Check sheet for the modelled part. Datum: model origin and axes. Units: mm. Face numbers are marked on the shaded views. A direction names the side the tool comes from. Give positions to 0.01 mm unless a question says otherwise; leave off trailing zeros. Write each loop counter-clockwise with the first axis right and the second up, starting at its lowest first coordinate (ties: lowest second). Pieces come first, ordered by that corner, then holes. Notation, with made-up numbers: (49.5, -1) - (59.5, -1) arc R15 cw to (59.5, 27) - close; hole circle Ø1 at (-23, 80). An arc over 180 degrees is marked (long way). Return JSON: item names as keys, results as strings. Group by question number.
```python
from build123d import *

# Parameters (mm, degrees)
SKETCH1_W           = 82.55
SKETCH1_H           = 22.225
BOSS_EXTRUDE1_DEPTH = 6.35
SKETCH3_W           = 3.175
SKETCH3_H           = 25.4
BOSS_EXTRUDE2_DEPTH = 22.225
CUT_EXTRUDE3_START  = 3.175
SKETCH2_W           = 38.1
SKETCH2_H           = 3.175
CUT_EXTRUDE3_DEPTH  = 50.972604439


with BuildPart() as part:
    # Sketch1 → Boss-Extrude1 (new body)
    with BuildSketch(Plane.XY):
        Rectangle(SKETCH1_W, SKETCH1_H)
    extrude(amount=BOSS_EXTRUDE1_DEPTH)

    # Sketch3 → Boss-Extrude2 (add)
    with BuildSketch(Plane(origin=(0, 11.1125, 0), x_dir=(1, 0, 0), z_dir=(0, 1, 0))):
        with Locations((-19.05, 6.35)):
            Rectangle(SKETCH3_W, SKETCH3_H)
        with Locations((19.05, 6.35)):
            Rectangle(SKETCH3_W, SKETCH3_H)
    extrude(amount=-BOSS_EXTRUDE2_DEPTH)

    # Sketch2 → Cut-Extrude3 (cut, through all)
    with BuildSketch(Plane.XY.offset(CUT_EXTRUDE3_START)):
        Rectangle(SKETCH2_W, SKETCH2_H)
    extrude(amount=-CUT_EXTRUDE3_DEPTH, mode=Mode.SUBTRACT)


solid = part.part
```
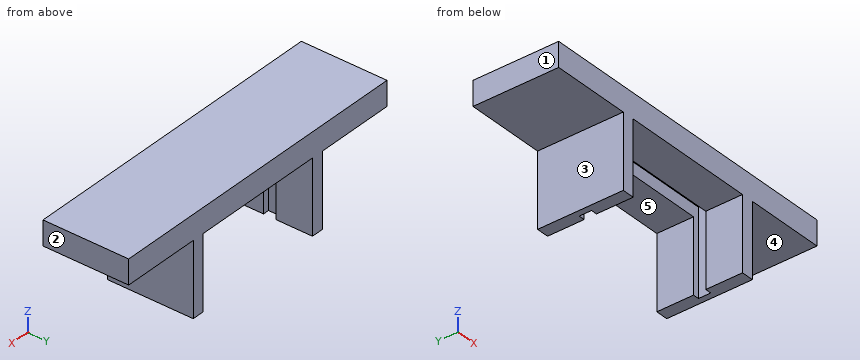
Item 1: Section check D-D on x = 29. Record the cut outline in (y, z).
Item 2: Section check A-A on z = -1. Record the cut outline in (x, y), plus the area to 3 significant figures.
Item 3: Depth check by flat-ended pin: pin 1 (3 mm diameter, centred on y = -8, z = -13, fed in from -X); pin 2 (12 mm diameter, centred on x = -30.5, z = -14, fed in from -Y); pin 3 (12 mm diameter, centred on x = -10.5, y = 3.5, fed in from -Z); pin 4 (5 mm diameter, centred on y = -6.5, z = -10.5, fed in from +X). Enter the tip coordinate at first touch or a pass-through.
Item 4: Material ranges on line 1 along X through (y, z) = (3.5, -11.5); line 2 along Y through (x, z) = (16, 1); line 3 along X through (y, z) = (-0.75, -7.5), recorded low to high. Write a range as from..to.
Item 5: Access from +Z, -Z, +X, -X, +Y, -Y to the whole of each face (thin tool, end or side, straight path). Record for the marked faces 1, 2, 3, 4 and 5.
Reply:
{
 "1": {"outline": "(-11.11, 0) - (11.11, 0) - (11.11, 6.35) - (-11.11, 6.35) - close"},
 "2": {"outline": "(-20.64, -11.11) - (-17.46, -11.11) - (-17.46, -1.59) - (-19.05, -1.59) - (-19.05, 1.59) - (-17.46, 1.59) - (-17.46, 11.11) - (-20.64, 11.11) - close; (17.46, -11.11) - (20.64, -11.11) - (20.64, 11.11) - (17.46, 11.11) - (17.46, 1.59) - (19.05, 1.59) - (19.05, -1.59) - (17.46, -1.59) - close", "area": "131 mm²"},
 "3": {"pin 1": "x = -20.64", "pin 2": "through", "pin 3": "z = 0", "pin 4": "x = 20.64"},
 "4": {"line 1": "-20.64..-17.46, 17.46..20.64", "line 2": "-11.11..-1.59, 1.59..11.11", "line 3": "-20.64..-19.05, 19.05..20.64"},
 "5": {"face 1": "+Z, -Z, -X, +Y, -Y", "face 2": "+Z, -Z, +X, +Y, -Y", "face 3": "-Z, -X, +Y, -Y", "face 4": "-Z, +X, +Y, -Y", "face 5": "-Z, +Y, -Y"}
}
